Drawing for the job (mm, zero at the part's lowest x, y, z). Give positions to 0.01 mm unless a question says otherwise; leave off trailing zeros. Order: outer loops, then holes, each group sorted by start corner. A loop starts at its lowest first (then second) coordinate and runs counter-clockwise, first axis right, second up. Notation, with made-up numbers: (11, 86.25) -> (35, 86.25) arc R17 ccw to (35, 98.25) -> close; hole circle Ø8 at (79, -6.5). An arc over 180 degrees is marked (long way). Use one line per item in the form item = value. Start each with the question number.
1) Probe line 1 (X direction, y = 1.6, z = 13.5) (1 decimal); line 2 (Y direction, x = 0.3, z = 14.5) (1 decimal); line 3 (Y direction, x = 1.3, z = 1.75). List the from-to ranges inside material, lowest first.
2) Drop a flat-ended pin along its axis: P1, Ø1, axis at y = 1, z = 18, coming from the -X side. Give the stop position or say it passes through.
3) Cut at A-A, the plane z = 22. Give the cut face in (x, y) (1 decimal).
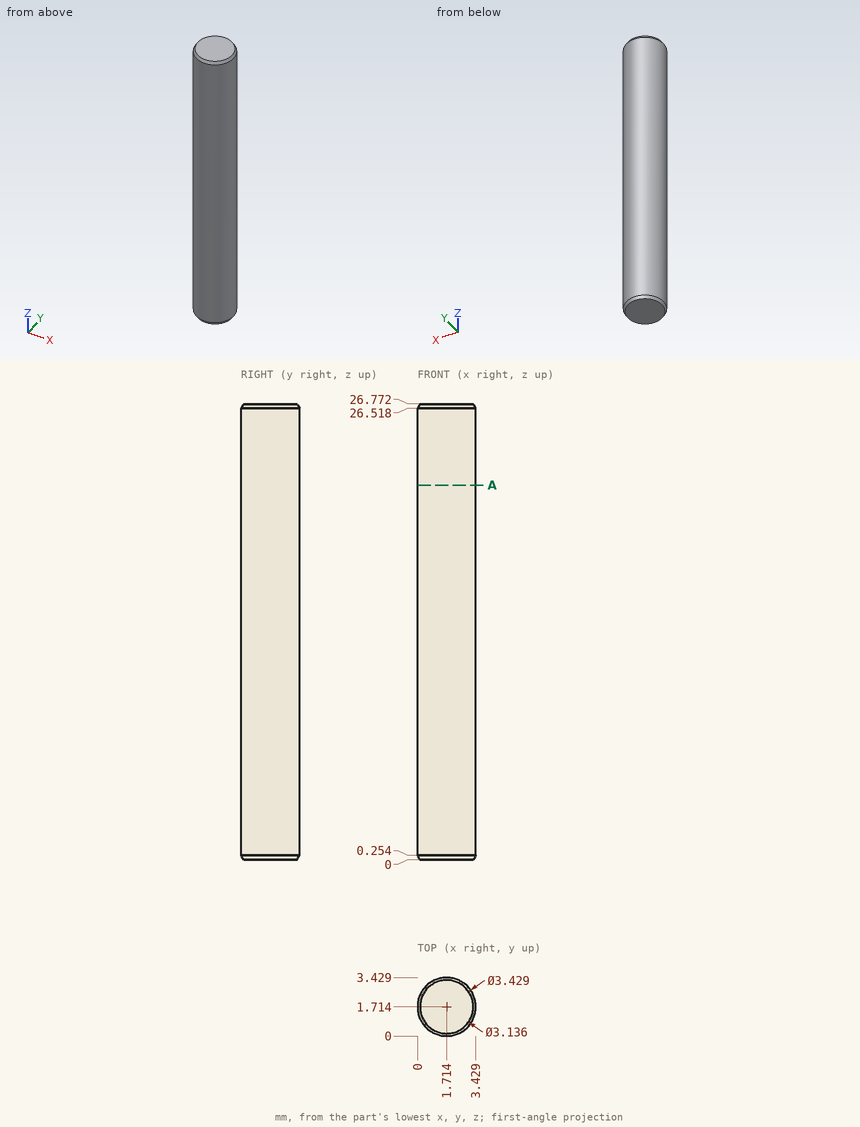
Result:
q1.line_1 = 0 to 3.4
q1.line_2 = 0.7 to 2.7
q1.line_3 = 0.05 to 3.38
q2.P1 = 0.01
q3.outline = circle Ø3.4 at (1.7, 1.7)
